Source: CAD feature listing. Evaluate the final solid. Frame: model axes, mm. Give positions to 0.01 mm unless a question says otherwise; leave off trailing zeros. Order: outer loops, then holes, each group sorted by start corner. A loop starts at its lowest first (then second) coordinate and runs counter-clockwise, first axis right, second up. Notation, with made-up numbers: M -24,63.5 L 9,63.5 A15 ccw 9,75.5 Z; hole C 11,53 d11. An arc over 180 degrees is marked long. Use CSV: the item, a comma, the result in double quotes. Start each with the question number.
1. Section query D-D, the plane z = -127.5. Return the cut outline in (x, y).
2. Section query B-B, the plane y = 5.25. State how many separate pieces and enclosed holes the cut face has, plus the area to 3 significant figures.
3. Section query C-C, the plane x = 51. Return the cut outline in (y, z), plus the area to 3 significant figures.
4. Line query: line 1 along X through (y, z) = (2.5, -166); line 2 along X through (y, z) = (5, -102); line 3 along Z through (x, y) = (43, 5.75). Output: solid intervals per line, ascending. Write a range as [from, to].
5. Section query A-A, the plane x = -25. Return the cut outline in (y, z), plus the area to 3 significant figures.
Autodesk Inventor part; units mm, degrees
ref_plane "YZ Plane" through (0, 0, 0) normal (1, 0, 0) x (0, 1, 0)
ref_plane "XZ Plane" through (0, 0, 0) normal (0, 1, 0) x (-1, 0, 0)
ref_plane "XY Plane" through (0, 0, 0) normal (0, 0, 1) x (1, 0, 0)
sketch "Sketch1" plane through (0, 0, 0) normal (0, 1, 0) x (-1, 0, 0)
  arc A0 (-69, -145.9) -> (-66, -148.9) centre (-66, -145.9) ccw
  line L0 (-64.5, -148.9) -> (-66, -148.9)
  arc A1 (-68, -155.4) -> (-72, -155.4) centre (-70, -155.4) ccw
  line L1 (-68, -155.4) -> (-68, -158.4)
  line L2 (-72, -158.4) -> (-72, -155.4)
  arc A2 (-72, -158.4) -> (-68, -158.4) centre (-70, -158.4) ccw
  line L3 (-61.5, -162) -> (-61.5, -151.9)
  arc A3 (-66.25, -165.2) -> (-69.75, -165.2) centre (-68, -165.2) ccw
  line L4 (-66.25, -165.2) -> (-66.25, -168.2)
  line L5 (-69.75, -168.2) -> (-69.75, -165.2)
  arc A4 (-69.75, -168.2) -> (-66.25, -168.2) centre (-68, -168.2) ccw
  arc A5 (-61.5, -151.9) -> (-64.5, -148.9) centre (-64.5, -151.9) ccw
  arc A6 (61.5, -94.6) -> (58.5, -91.6) centre (58.5, -94.6) ccw
  line L6 (61.5, -94.6) -> (61.5, -107.7)
  line L7 (66.25, -94.4) -> (66.25, -91.4)
  arc A7 (69.75, -91.4) -> (66.25, -91.4) centre (68, -91.4) ccw
  line L8 (69.75, -91.4) -> (69.75, -94.4)
  arc A8 (66.25, -94.4) -> (69.75, -94.4) centre (68, -94.4) ccw
  arc A9 (71.75, -101.2) -> (68.25, -101.2) centre (70, -101.2) ccw
  line L9 (71.75, -101.2) -> (71.75, -104.2)
  arc A10 (68.25, -104.2) -> (71.75, -104.2) centre (70, -104.2) ccw
  arc A11 (61.5, -107.7) -> (64.5, -110.7) centre (64.5, -107.7) ccw
  line L10 (64.5, -110.7) -> (66, -110.7)
  arc A12 (69, -113.7) -> (66, -110.7) centre (66, -113.7) ccw
  line L11 (69, -113.7) -> (69, -158.4)
  line L12 (68.25, -104.2) -> (68.25, -101.2)
  arc A13 (66, -161.4) -> (69, -158.4) centre (66, -158.4) ccw
  arc A14 (71.75, -165.2) -> (68.25, -165.2) centre (70, -165.2) ccw
  line L13 (71.75, -165.2) -> (71.75, -168.2)
  arc A15 (68.25, -168.2) -> (71.75, -168.2) centre (70, -168.2) ccw
  line L14 (68.25, -168.2) -> (68.25, -165.2)
  line L15 (66, -161.4) -> (39.9991, -161.4)
  arc A16 (45.75, -165.4) -> (42.25, -165.4) centre (44, -165.4) ccw
  arc A17 (39.9991, -161.4) -> (37.2495, -163.2) centre (39.9991, -164.4) ccw
  line L16 (45.75, -165.4) -> (45.75, -168.4)
  arc A18 (34.5, -165) -> (37.2495, -163.2) centre (34.5, -162) ccw
  line L17 (42.25, -168.4) -> (42.25, -165.4)
  arc A19 (42.25, -168.4) -> (45.75, -168.4) centre (44, -168.4) ccw
  line L18 (34.5, -165) -> (-58.5, -165)
  arc A20 (-61.5, -162) -> (-58.5, -165) centre (-58.5, -162) ccw
  line L19 (-66, -98.4) -> (-40.5, -98.4)
  arc A21 (-71.75, -94.4) -> (-68.25, -94.4) centre (-70, -94.4) ccw
  arc A22 (-68.25, -91.4) -> (-71.75, -91.4) centre (-70, -91.4) ccw
  line L20 (-71.75, -94.4) -> (-71.75, -91.4)
  line L21 (-68.25, -91.4) -> (-68.25, -94.4)
  line L22 (-69, -145.9) -> (-69, -101.4)
  arc A23 (-66, -98.4) -> (-69, -101.4) centre (-66, -101.4) ccw
  line L23 (-45.75, -94.2) -> (-45.75, -91.2)
  arc A24 (-42.25, -91.2) -> (-45.75, -91.2) centre (-44, -91.2) ccw
  line L24 (-42.25, -91.2) -> (-42.25, -94.2)
  arc A25 (-45.75, -94.2) -> (-42.25, -94.2) centre (-44, -94.2) ccw
  line L25 (-34.5, -91.6) -> (58.5, -91.6)
  arc A26 (-34.5, -91.6) -> (-37.5, -94.6) centre (-34.5, -94.6) ccw
  line L26 (-37.5, -95.4) -> (-37.5, -94.6)
  arc A27 (-40.5, -98.4) -> (-37.5, -95.4) centre (-40.5, -95.4) ccw
  line L27 (74.75, -86.45) -> (-74.75, -86.45)
  line L28 (-74.75, -86.45) -> (-74.75, -173.15)
  line L29 (-74.75, -173.15) -> (74.75, -173.15)
  line L30 (74.75, -173.15) -> (74.75, -86.45)
  point P0 (0, 0)
  dimension "d0" = 1.75
  dimension "d1" = 3
  dimension "d2" = 2
  dimension "d3" = 2
  dimension "d4" = 2.75
  dimension "d5" = 10.25
  dimension "d6" = 26
  dimension "d7" = 109.25
  dimension "d8" = 114
  dimension "d9" = 133.25
  dimension "d10" = 138
  dimension "d11" = 139.75
  dimension "d12" = 140
  dimension "d13" = 140.75
  dimension "d14" = 50.7
  dimension "d15" = 19.1
  dimension "d16" = 54.3
  dimension "d17" = 12.3
  dimension "d18" = 38.2
  dimension "d19" = 9.5
  dimension "d20" = 6.5
  dimension "d21" = 54.5
  dimension "d22" = 57.5
  dimension "d23" = 19.3
  dimension "d24" = 16.3
  dimension "d25" = 54.7
  dimension "d26" = 57.7
  dimension "d27" = 31.7509
  dimension "d28" = 19.5
  dimension "d29" = 16.5
  dimension "d30" = 54.5
  dimension "d31" = 44.7
  dimension "d32" = 137.75
  dimension "d33" = 57.5
  dimension "d34" = 16.3
  dimension "d35" = 139
  dimension "d36" = 19.3
  dimension "d37" = 139
  dimension "d38" = 47.7
  dimension "d40" = 3
  dimension "d41" = 3
  dimension "d42" = 3
  dimension "d43" = 3
extrude "Extrusion1" add sketch "Sketch1" along normal blind 9
fillet "Fillet1" radius 3 4 edges at (-74.75, 4.5, -86.45) (-74.75, 4.5, -173.15) (74.75, 4.5, -173.15) (74.75, 4.5, -86.45)
sketch "Sketch2" plane through (0, 9, 0) normal (0, 1, 0) x (1, 0, 0)
  line L0 (-69, 113.7) -> (-69, 158.4)
  line L1 (-74.75, 170.15) -> (-74.75, 89.45)
  arc A0 (-66, 161.4) -> (-69, 158.4) centre (-66, 158.4) ccw
  arc A1 (-70.5, 156.9) -> (-69, 158.4) centre (-70.5, 158.4) ccw
  arc A2 (-74.75, 158.4) -> (-73.25, 156.9) centre (-73.25, 158.4) ccw
  line L2 (-73.25, 156.9) -> (-70.5, 156.9)
  line L3 (-73.25, 115.2) -> (-70.5, 115.2)
  arc A3 (-73.25, 115.2) -> (-74.75, 113.7) centre (-73.25, 113.7) ccw
  arc A4 (-69, 113.7) -> (-70.5, 115.2) centre (-70.5, 113.7) ccw
  point P0 (0, 0)
  dimension "d50" = 3
  dimension "d51" = 3
extrude "Extrusion3" cut sketch "Sketch2" against normal up to surface (9 mm away)
properties part number "psu_spacer"
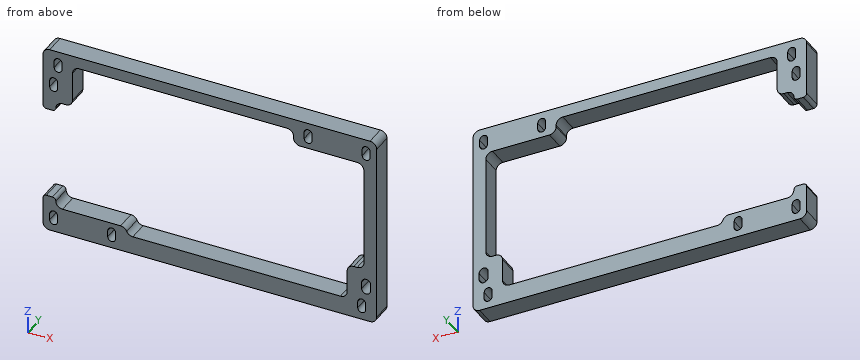
Result set:
1,outline,"M 69,0 L 74.75,0 L 74.75,9 L 69,9 Z"
2,separate pieces,"1"
2,enclosed holes,"8"
2,area,"3,020 mm2"
3,outline,"M 0,-173.15 L 9,-173.15 L 9,-165 L 0,-165 Z; M 0,-98.4 L 9,-98.4 L 9,-86.45 L 0,-86.45 Z"
3,area,"181 mm2"
4,line 1,"[-74.75, -71.75], [-68.25, -45.75], [-42.25, 66.25], [69.75, 74.75]"
4,line 2,"[-74.75, -71.75], [-68.25, -61.5], [69, 74.75]"
4,line 3,"[-173.15, -165], [-98.4, -95.64], [-89.76, -86.45]"
5,outline,"M 0,-173.15 L 9,-173.15 L 9,-165 L 0,-165 Z; M 0,-91.6 L 9,-91.6 L 9,-86.45 L 0,-86.45 Z"
5,area,"120 mm2"
